```python
from build123d import *

# Parameters (mm, degrees)
SKETCH1_R               = 25
BOSS_EXTRUDE1_DEPTH     = 4
SKETCH2_R               = 1.713577746
CUT_EXTRUDE1_DEPTH      = 4
CUT_EXTRUDE2_DEPTH      = 2
SKETCH4_R               = 12.5
SKETCH4_R_2             = 2.5
BOSS_EXTRUDE2_DEPTH     = 10
SKETCH5_R               = 1.6
CUT_EXTRUDE3_DEPTH      = 12.5
SKETCH6_R               = 3.1
CUT_EXTRUDE4_DEPTH      = 6
FILLET1_R               = 1.5
SKETCH9_R               = 8.75
CUT_EXTRUDE6_DEPTH      = 3
SKETCH12_W              = 5.5
SKETCH12_H              = 2.5
CUT_EXTRUDE7_DEPTH      = 10
CUT_EXTRUDE8_DEPTH      = 10
CUT_EXTRUDE8_DEPTH_BACK = 2
SKETCH17_R              = 1.6
CUT_EXTRUDE9_DEPTH      = 30
CUT_EXTRUDE9_DEPTH_BACK = 2
SKETCH18_R              = 1.6
CUT_EXTRUDE10_START     = -3
SKETCH20_R              = 3.1
CUT_EXTRUDE10_DEPTH     = 4
CUT_EXTRUDE11_START     = -3
SKETCH21_R              = 3.1
CUT_EXTRUDE11_DEPTH     = 4


with BuildPart() as part:
    # Sketch1 → Boss-Extrude1 (new body)
    with BuildSketch(Plane.XY):
        Circle(SKETCH1_R)
    extrude(amount=BOSS_EXTRUDE1_DEPTH)

    # Sketch2 → Cut-Extrude1 (cut)
    with BuildSketch(Plane(origin=(0, 0, 0), x_dir=(-1, 0, 0), z_dir=(0, 0, -1))):
        with Locations((0, 18.35)):
            Circle(SKETCH2_R)
        with Locations((15.891566159, 9.175)):
            Circle(SKETCH2_R)
        with Locations((15.891566159, -9.175)):
            Circle(SKETCH2_R)
        with Locations((0, -18.35)):
            Circle(SKETCH2_R)
        with Locations((-15.891566159, -9.175)):
            Circle(SKETCH2_R)
        with Locations((-15.891566159, 9.175)):
            Circle(SKETCH2_R)
    extrude(amount=-CUT_EXTRUDE1_DEPTH, mode=Mode.SUBTRACT)

    # Sketch3 → Cut-Extrude2 (cut)
    with BuildSketch(Plane(origin=(0, 0, 0), x_dir=(-1, 0, 0), z_dir=(0, 0, -1))):
        Polygon((13.870840217, 5.675), (17.912292102, 5.675), (19.933018044, 9.175), (17.912292102, 12.675), (13.870840217, 12.675), (11.850114275, 9.175), align=None)
        Polygon((4.041451884, 18.35), (2.020725942, 21.85), (-2.020725942, 21.85), (-4.041451884, 18.35), (-2.020725942, 14.85), (2.020725942, 14.85), align=None)
        Polygon((11.850114275, -9.175), (13.870840217, -12.675), (17.912292102, -12.675), (19.933018044, -9.175), (17.912292102, -5.675), (13.870840217, -5.675), align=None)
        Polygon((-2.020725942, -14.85), (-4.041451884, -18.35), (-2.020725942, -21.85), (2.020725942, -21.85), (4.041451884, -18.35), (2.020725942, -14.85), align=None)
        Polygon((-13.870840217, -5.675), (-17.912292102, -5.675), (-19.933018044, -9.175), (-17.912292102, -12.675), (-13.870840217, -12.675), (-11.850114275, -9.175), align=None)
        Polygon((-11.850114275, 9.175), (-13.870840217, 12.675), (-17.912292102, 12.675), (-19.933018044, 9.175), (-17.912292102, 5.675), (-13.870840217, 5.675), align=None)
    extrude(amount=-CUT_EXTRUDE2_DEPTH, mode=Mode.SUBTRACT)

    # Sketch4 → Boss-Extrude2 (add)
    with BuildSketch(Plane(origin=(0, 0, 0), x_dir=(-1, 0, 0), z_dir=(0, 0, -1))):
        with Locations(Location((0, 0, 0), (0, 0, 180))):
            Circle(SKETCH4_R)
        with Locations((0, 0.5)):
            Circle(SKETCH4_R_2, mode=Mode.SUBTRACT)
    extrude(amount=BOSS_EXTRUDE2_DEPTH)

    # Sketch5 → Cut-Extrude3 (cut)
    with BuildSketch(Plane(origin=(0, 12.5, 0), x_dir=(1, 0, 0), z_dir=(0, 1, 0))):
        with Locations(Location((0, 5, 0), (0, 0, 270))):
            Circle(SKETCH5_R)
    extrude(amount=-CUT_EXTRUDE3_DEPTH, mode=Mode.SUBTRACT)

    # Sketch6 → Cut-Extrude4 (cut)
    with BuildSketch(Plane(origin=(0, 12.5, 0), x_dir=(1, 0, 0), z_dir=(0, 1, 0))):
        with Locations(Location((0, 5, 0), (0, 0, 270))):
            Circle(SKETCH6_R)
    extrude(amount=-CUT_EXTRUDE4_DEPTH, mode=Mode.SUBTRACT)

    # Fillet1
    fillet1_edges = [part.edges().sort_by_distance(p)[0] for p in [
        (-12.5, 0, 0),
    ]]
    fillet(fillet1_edges, radius=FILLET1_R)

    # Sketch9 → Cut-Extrude6 (cut)
    with BuildSketch(Plane.XY.offset(4)):
        Circle(SKETCH9_R)
    extrude(amount=-CUT_EXTRUDE6_DEPTH, mode=Mode.SUBTRACT)

    # Sketch12 → Cut-Extrude7 (cut)
    with BuildSketch(Plane(origin=(0, 0, -10), x_dir=(-1, 0, 0), z_dir=(0, 0, -1))):
        Polygon((1.223076211, -3.88156986), (3.973076211, 0.88156986), (6.138139721, -0.36843014), (3.388139721, -5.13156986), align=None)
        with Locations((0, 3.25)):
            Rectangle(SKETCH12_W, SKETCH12_H)
        Polygon((-3.388139721, -5.13156986), (-1.223076211, -3.88156986), (-3.973076211, 0.88156986), (-6.138139721, -0.36843014), align=None)
    extrude(amount=-CUT_EXTRUDE7_DEPTH, mode=Mode.SUBTRACT)

    # Sketch17 → Cut-Extrude8 (cut, two sides: drawn at the far end of the back side and taken through both)
    with BuildSketch(Plane(origin=(2.598076211, -1.5, 0), x_dir=(0, 0, -1), z_dir=(0.8660254037844387, -0.4999999999999998, 0)).offset(-CUT_EXTRUDE8_DEPTH_BACK)):
        with Locations(Location((5, 0, 0), (0, 0, 90))):
            Circle(SKETCH17_R)
    extrude(amount=CUT_EXTRUDE8_DEPTH + CUT_EXTRUDE8_DEPTH_BACK, mode=Mode.SUBTRACT)

    # Sketch18 → Cut-Extrude9 (cut, two sides: drawn at the far end of the back side and taken through both)
    with BuildSketch(Plane(origin=(-2.598076211, -1.5, 0), x_dir=(0, 0, 1), z_dir=(-0.8660254037844388, -0.49999999999999983, 0)).offset(-CUT_EXTRUDE9_DEPTH_BACK)):
        with Locations(Location((-5, 0, 0), (0, 0, 90))):
            Circle(SKETCH18_R)
    extrude(amount=CUT_EXTRUDE9_DEPTH + CUT_EXTRUDE9_DEPTH_BACK, mode=Mode.SUBTRACT)

    # Sketch20 → Cut-Extrude10 (cut)
    with BuildSketch(Plane(origin=(-4.763139721, -2.75, 0), x_dir=(0, 0, -1), z_dir=(0.866025403784439, 0.4999999999999994, 0)).offset(CUT_EXTRUDE10_START)):
        with Locations(Location((5, 0, 0), (0, 0, 90))):
            Circle(SKETCH20_R)
    extrude(amount=-CUT_EXTRUDE10_DEPTH, mode=Mode.SUBTRACT)

    # Sketch21 → Cut-Extrude11 (cut)
    with BuildSketch(Plane(origin=(4.763139721, -2.75, 0), x_dir=(0, 0, 1), z_dir=(-0.866025403784439, 0.4999999999999994, 0)).offset(CUT_EXTRUDE11_START)):
        with Locations(Location((-5, 0, 0), (0, 0, 270))):
            Circle(SKETCH21_R)
    extrude(amount=-CUT_EXTRUDE11_DEPTH, mode=Mode.SUBTRACT)


solid = part.part
```
CAD build for the part. Positions are in the model's coordinates, mm. A direction names the side the tool comes from. Round coordinates to 2 decimals unless told otherwise and drop trailing zeros. Order: outer loops, then holes, each group sorted by start corner. A loop starts at its lowest first (then second) coordinate and runs counter-clockwise, first axis right, second up. Notation, with made-up numbers: (70.5, 69.5) - (125.5, 69.5) arc R10 cw to (125.5, 74.5) - close; hole circle Ø6 at (-8.75, 51.25). An arc over 180 degrees is marked (long way). Answer in a Markdown table with one row per item. Add a question column.
(1) 3-axis set-ups, long thin cutter, end or side, ignore diameter. For faces 1 (the face through (0, -11, 4)), 2 (the face through (5.7, -1.13, -5.07)), 3 (the face through (0, 0, 1)): which of +Z, -Z, +X, -X, +Y, -Y reach the whole face in a straight line?
(2) Band-saw the part on B-B on z = -4.25. Count the separate pieces of the cut face and the enclosed holes in it, and give its area (3 significant figures).
(3) Mould opens along Y. For faces 4 (the face through (-0.97, 5.51, -6.27)), 5 (the face through (-16, 5.675, 1)) say: +Y half, -Y half, draft (parallel to the pull), parting line (faces both ways), or undercut.
(4) Drop flat-ended pins along their axis: pin 1 Ø2 at (x, z) = (-15, 1.5) entering from +Y; pin 2 Ø1 at (x, z) = (15, 1.5) entering from +Y; pin 3 Ø7.5 at (x, y) = (-2, -19) entering from -Z. Give the stop position or say it passes through.
(5) Probe L1, parallel to Y at x = 0, z = 2.4; L2, parallel to Y at x = 17, z = 3; L3, parallel to Z at x = 13, y = -17.5. List the from-to ranges inside material, lowest first. Write a range as [from, to].
(6) Band-saw the part on A-A on z = -8.75. List the corners of the cut face in (x, y).
Data:
| question | item | result |
|---|---|---|
| 1 | face 1 | +Z, +X, -X, +Y, -Y |
| 1 | face 2 | -Z |
| 1 | face 3 | +Z |
| 2 | separate pieces | 3 |
| 2 | enclosed holes | 0 |
| 2 | area | 323 mm^2 |
| 3 | face 4 | draft |
| 3 | face 5 | undercut |
| 4 | pin 1 | stops at y = 20.71 |
| 4 | pin 2 | stops at y = 20.37 |
| 4 | pin 3 | stops at z = 0 |
| 5 | L1 | y = [-25, -20.06], [-16.64, -8.75], [8.75, 16.64], [20.06, 25] |
| 5 | L2 | y = [-18.33, -10.48], [-7.87, 7.87], [10.48, 18.33] |
| 5 | L3 | z = [0, 4] |
| 6 | outline | circle Ø25 at (0, 0); hole (-6.14, -0.37) - (-3.39, -5.13) - (-1.22, -3.88) - (-3.97, 0.88) - close; hole (-2.75, 2) - (-2, 2) arc R2.5 ccw (long way) to (2, 2) - (2.75, 2) - (2.75, 4.5) - (-2.75, 4.5) - close; hole (1.22, -3.88) - (3.39, -5.13) - (6.14, -0.37) - (3.97, 0.88) - close |
